```python
from build123d import *

# Parameters (mm, degrees)
F4_DEPTH  = 9
F6_DEPTH  = 2
F8_DEPTH  = 2
F9_W      = 9
F9_H      = 2
F10_DEPTH = 2
F11_W     = 17
F11_H     = 2
F12_DEPTH = 4


# Not quite as in the source:
# - a pattern or mirror of a feature is missing from the dataset's text; its kind, count and spacing are read off the source's solid


with BuildPart() as f4:
    # F3 (on plane+point) → F4 (new body, through all)
    with BuildSketch(Plane.YZ.offset(4.5)):
        Polygon((4.5, 0), (6.5, 0), (6.5, 4), (-5.5, 10.9282032303), (-5.5, 8.9282032303), (4.5, 3.1547005384), align=None)
    extrude(amount=-F4_DEPTH)

    # F5 (on face) → F6 (join)
    with BuildSketch(Plane.YZ.offset(4.5)):
        Polygon((6.5, 4), (-5.5, 10.9282032303), (-5.5, 0), (6.5, 0), align=None)
    f6 = extrude(amount=F6_DEPTH)

    # F6_copies: F6 across plane
    add(f6.mirror(Plane(origin=(0, 0, 0), x_dir=(0, 0, -1), z_dir=(-1, 0, 0))))

    # F7 (on Top) → F8 (join)
    with BuildSketch(Plane.XY):
        Polygon((4.5, 8.5), (4.5, 6.5), (6.5, 6.5), (6.5, -5.5), (8.5, -5.5), (8.5, 8.5), align=None)
    f8 = extrude(amount=F8_DEPTH)

    # F8_copies: F8 across plane
    add(f8.mirror(Plane(origin=(0, 0, 0), x_dir=(0, 0, -1), z_dir=(-1, 0, 0))))

    # F9 (on face) → F10 (cut, through all)
    with BuildSketch(Plane(origin=(0, 6.5, 0), x_dir=(-1, 0, 0), z_dir=(0, 1, 0))):
        with Locations((0, 1)):
            Rectangle(F9_W, F9_H)
    extrude(amount=-F10_DEPTH, mode=Mode.SUBTRACT)

    # F11 (on Top) → F12 (join)
    with BuildSketch(Plane.XY):
        with Locations((0, 9.5)):
            Rectangle(F11_W, F11_H)
    extrude(amount=F12_DEPTH)


solid = f4.part
```
Design review of the part built by this model. Coordinates are the model's own, in mm. A direction names the side the tool comes from. Give positions to 0.01 mm unless a question says otherwise; leave off trailing zeros. Order: outer loops, then holes, each group sorted by start corner. A loop starts at its lowest first (then second) coordinate and runs counter-clockwise, first axis right, second up. Notation, with made-up numbers: (19, -34) - (36, -34) arc R11 cw to (36, -21) - close; hole circle Ø10 at (21.5, -23.5). An arc over 180 degrees is marked (long way). Use a Markdown table: item, result. Add a question column.
(1) Add section A-A on x = 2.75. Give the boundary of the cut face in (y, z).
(2) Machinability: for faces 4 (the face through (0, 8.5, 2)), 5 (the face through (0, 6.5, 3)), 6 (the face through (6.5, -1, 6)), 7 (the face through (0, 10, 4)), 8 (the face through (-4.5, 0, 3)), which of the approach directions +Z, -Z, +X, -X, +Y, -Y give a long, thin tool a straight path to every point of the face, cutting with its end or side? Answer none if there is none.
(3) Add section B-B on y = 7.5. Give the boundary of the cut face in (x, z).
(4) Mouldability with a two-part tool opening along X and no side actions: class faces 1 (the face through (0.09, 0.58, 7.42)), 2 (the face through (4.5, 0, 3)), 3 (the face through (-8.5, 2, 1)) as +X half, -X half, draft (parallel to the pull), parting line (faces both ways), or undercut.
(5) Wall thickness on probe 1 along Y at (x, z) = (-2.25, 2.5); probe 2 along X at (y, z) = (4.25, 2.75); probe 3 along X at (y, z) = (7.5, 1.25): over which ranges is each line inside the solid? List them lowest first. Write a range as [from, to].
(6) Clearance check with flat-ended pins moving along their axes: P1, Ø0.9, axis at x = -1.5, z = 2.5, coming from the -Y side; P2, Ø1.6, axis at x = 0.5, y = 5, coming from the -Z side; P3, Ø2, axis at x = -0.5, y = 9.5, coming from the +Z side. State where each tip first meets the part, or that it passes through.
(7) Add section C-C on z = 2.75. Give the boundary of the cut face in (x, y).
(8) Add section D-D on x = -5. Give the boundary of the cut face in (y, z).
Report:
| question | item | result |
|---|---|---|
| 1 | outline | (-5.5, 8.93) - (4.5, 3.15) - (4.5, 2) - (6.5, 2) - (6.5, 4) - (-5.5, 10.93) - close; (8.5, 0) - (10.5, 0) - (10.5, 4) - (8.5, 4) - close |
| 2 | face 4 | +Z |
| 2 | face 5 | +Z, +X, -X |
| 2 | face 6 | +Z, +X, -Y |
| 2 | face 7 | +Z, +X, -X, +Y |
| 2 | face 8 | -Z, -Y |
| 3 | outline | (-8.5, 0) - (-4.5, 0) - (-4.5, 2) - (-8.5, 2) - close; (4.5, 0) - (8.5, 0) - (8.5, 2) - (4.5, 2) - close |
| 4 | face 1 | draft |
| 4 | face 2 | undercut |
| 4 | face 3 | -X half |
| 5 | probe 1 | y = [4.5, 6.5], [8.5, 10.5] |
| 5 | probe 2 | x = [-6.5, -4.5], [4.5, 6.5] |
| 5 | probe 3 | x = [-8.5, -4.5], [4.5, 8.5] |
| 6 | P1 | stops at y = 4.5 |
| 6 | P2 | stops at z = 2 |
| 6 | P3 | stops at z = 4 |
| 7 | outline | (-8.5, 8.5) - (8.5, 8.5) - (8.5, 10.5) - (-8.5, 10.5) - close; (-6.5, -5.5) - (-4.5, -5.5) - (-4.5, 4.5) - (4.5, 4.5) - (4.5, -5.5) - (6.5, -5.5) - (6.5, 6.5) - (-6.5, 6.5) - close |
| 8 | outline | (-5.5, 0) - (10.5, 0) - (10.5, 4) - (8.5, 4) - (8.5, 2) - (6.5, 2) - (6.5, 4) - (-5.5, 10.93) - close |
